Work out the finished part from the listing and answer in its coordinate system (mm). Face numbers are marked on the shaded views. Coordinates: 2 decimals unless noted, no trailing zeros. Loops run counter-clockwise (first coordinate to the right, second up) from the corner with the lowest first, then second, coordinate; pieces in that order, holes last. Notation, with made-up numbers: (64.25, 83.25) -> (98.25, 83.25) arc R17 cw to (98.25, 88.25) -> close; hole circle Ø1 at (56, 21). An arc over 180 degrees is marked (long way). Use a Markdown table: item, result.
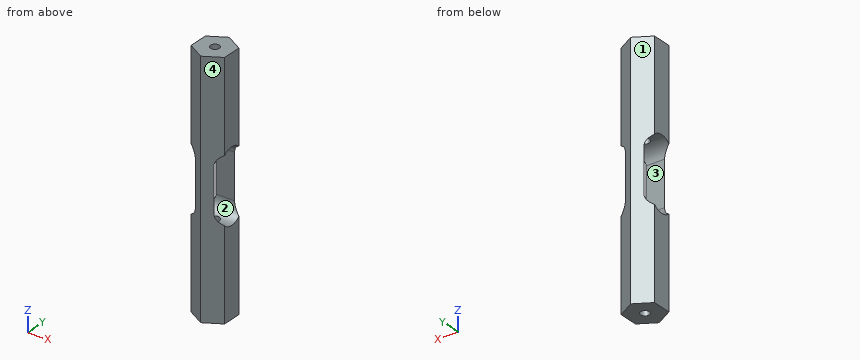
from build123d import *

# Parameters (mm, degrees)
BOSS_EXTRUDE1_DEPTH     = 34.925
CUT_EXTRUDE4_DEPTH      = 36.674625524
CUT_EXTRUDE4_DEPTH_BACK = 36.674625524
CUT_EXTRUDE5_DEPTH      = 36.674625524
CUT_EXTRUDE5_DEPTH_BACK = 36.674625524
SKETCH6_R               = 1.25


with BuildPart() as part:
    # Sketch1 → Boss-Extrude1 (new, symmetric)
    with BuildSketch(Plane.XY):
        Polygon((0, 5.499261314), (-4.7625, 2.749630657), (-4.7625, -2.749630657), (0, -5.499261314), (4.7625, -2.749630657), (4.7625, 2.749630657), align=None)
    extrude(amount=BOSS_EXTRUDE1_DEPTH, both=True)

    # Sketch5 → Cut-Extrude4 (cut, two sides: drawn at the far end of the back side and taken through both)
    with BuildSketch(Plane(origin=(0, 0, 0), x_dir=(0, 0, -1), z_dir=(1, 0, 0)).offset(-CUT_EXTRUDE4_DEPTH_BACK)):
        with BuildLine():
            Line((-6.35, 3.96875), (6.35, 3.96875))
            ThreePointArc((6.35, 3.96875), (10.31875, 0), (6.35, -3.96875))
            Line((6.35, -3.96875), (-6.35, -3.96875))
            ThreePointArc((-6.35, -3.96875), (-10.31875, 0), (-6.35, 3.96875))
        make_face()
    extrude(amount=CUT_EXTRUDE4_DEPTH + CUT_EXTRUDE4_DEPTH_BACK, mode=Mode.SUBTRACT)

    # Sketch6 → Cut-Extrude5 (cut, two sides: drawn at the far end of the back side and taken through both)
    with BuildSketch(Plane.XY.offset(-CUT_EXTRUDE5_DEPTH_BACK)):
        Circle(SKETCH6_R)
    extrude(amount=CUT_EXTRUDE5_DEPTH + CUT_EXTRUDE5_DEPTH_BACK, mode=Mode.SUBTRACT)


solid = part.part
Q1. Given pin 1 Ø2 at (y, z) = (-3, -0.5) entering from +X; pin 2 Ø5 at (x, z) = (3, -12) entering from -Y; pin 3 Ø1.6 at (x, z) = (1.5, 2.5) entering from -Y; pin 4 Ø3 at (x, y) = (0, 0) entering from -Z (3 decimals), each flat-ended and moving along its own axis, determine where each tip first touches the part or whether it passes through.
Solved:
| item | result |
|---|---|
| pin 1 | x = 2.65 |
| pin 2 | y = -5.21 |
| pin 3 | y = -5.1 |
| pin 4 | z = -34.925 |
Q2. Consider line 1 (Y direction, x = 0, z = 21.75); line 2 (X direction, y = 0, z = -20); line 3 (Z direction, x = -2.75, y = 0) (3 decimals). Determine where each line is inside the solid, lowest interval first. Write a range as [from, to].
Solved:
| item | result |
|---|---|
| line 1 | [-5.5, -1.25], [1.25, 5.5] |
| line 2 | [-4.76, -1.25], [1.25, 4.76] |
| line 3 | [-34.925, -10.319], [10.319, 34.925] |
Q3. Section A-A on z = 19 is taken. Determine the outline of the cut face in (x, y).
Solved:
| item | result |
|---|---|
| outline | (-4.76, -2.75) -> (0, -5.5) -> (4.76, -2.75) -> (4.76, 2.75) -> (0, 5.5) -> (-4.76, 2.75) -> close; hole circle Ø2.5 at (0, 0) |
Q4. Determine the mould class of the marked faces 1, 2, 3 and 4 for opening direction Y: pulls with the +Y half, pulls with the -Y half, needs draft (parallel to the pull), parting line crosses it, or undercut.
Solved:
| item | result |
|---|---|
| face 1 | pulls with the +Y half |
| face 2 | undercut |
| face 3 | undercut |
| face 4 | pulls with the -Y half |
